Part print with two shaded views. Sizes in mm from the minimum x, y, z corner. A direction names the side the tool comes from. Round coordinates to 2 decimals unless told otherwise and drop trailing zeros. Write each loop counter-clockwise with the first axis right and the second up, starting at its lowest first coordinate (ties: lowest second). Pieces come first, ordered by that corner, then holes.
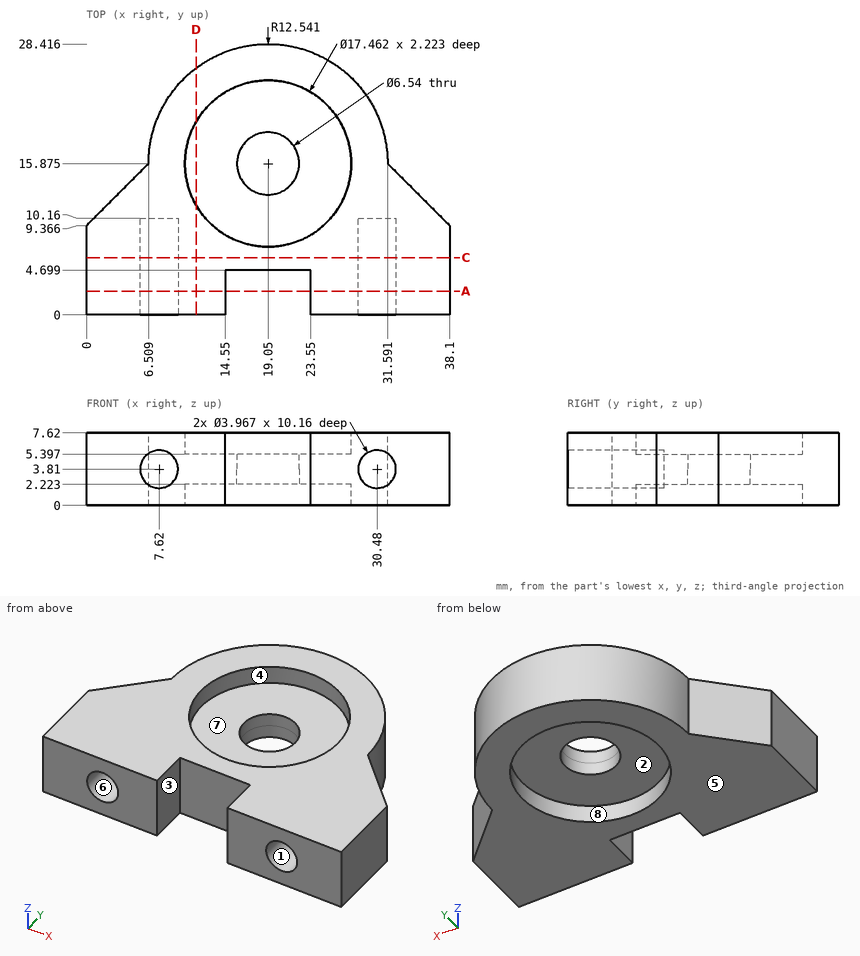
Q1. Drop flat-ended pins along their axis: pin 1 (1.5 mm diameter, centred on x = 24, z = 6, fed in from +Y); pin 2 (3.5 mm diameter, centred on x = 30.48, z = 3.81, fed in from -Y); pin 3 (5 mm diameter, centred on x = 21.5, y = 11, fed in from +Z); pin 4 (14 mm diameter, centred on x = 22, y = 15, fed in from -Z). Give the stop position or say it passes through.
Values follow:
pin 1: stops at y = 27.69
pin 2: stops at y = 10.16
pin 3: stops at z = 5.4
pin 4: stops at z = 0
Q2. Cut at D-D on x = 11.5. Write the cut outline in (y, z), plus the area to 3 significant figures.
Values follow:
outline: (0, 0) - (11.49, 0) - (11.49, 2.22) - (20.26, 2.22) - (20.26, 0) - (25.89, 0) - (25.89, 7.62) - (20.26, 7.62) - (20.26, 5.4) - (11.49, 5.4) - (11.49, 7.62) - (0, 7.62) - close
area: 158 mm2
Q3. Wall check: L1, parallel to X at y = 6.75, z = 3.81; L2, parallel to Z at x = 7.62, y = 3.75; L3, parallel to Y at x = 19.05, z = 4.85 (1 decimal). Give the ranges that are in metal, low to high.
Values follow:
L1: x = 0 to 5.64, 9.6 to 28.5, 32.46 to 38.1
L2: z = 0 to 1.83, 5.79 to 7.62
L3: y = 4.7 to 12.6, 19.1 to 28.4
Q4. Mould opens along Z. For the marked faces 5, 6, 7 and 8 say: +Z half, -Z half, draft (parallel to the pull), parting line (faces both ways), or undercut.
Values follow:
face 5: -Z half
face 6: undercut
face 7: +Z half
face 8: draft
Q5. Cut at C-C on y = 6. Write the cut outline in (x, z).
Values follow:
outline: (0, 0) - (38.1, 0) - (38.1, 7.62) - (0, 7.62) - close; hole circle Ø3.97 at (7.62, 3.81); hole circle Ø3.97 at (30.48, 3.81)
Q6. Which spindle directions (+Z, -Z, +X, -X, +Y, -Y) get a long thin tool onto all of the face, cutting with end or side? Do the marked faces 1, 2, 3 and 4. Say none if no direction does.
Values follow:
face 1: -Y
face 2: -Z
face 3: +Z, -Z, -Y
face 4: +Z
Q7. Cut at A-A on y = 2.5. Write the cut outline in (x, z), plus the area to 3 significant figures.
Values follow:
outline: (0, 0) - (14.55, 0) - (14.55, 7.62) - (0, 7.62) - close; (23.55, 0) - (38.1, 0) - (38.1, 7.62) - (23.55, 7.62) - close; hole circle Ø3.97 at (7.62, 3.81); hole circle Ø3.97 at (30.48, 3.81)
area: 197 mm2
